```python
from build123d import *

# Parameters (mm, degrees)
F0_W     = 100
F0_H     = 100
F1_DEPTH = 10
F2_SIZE  = 12
F4_D     = 9.5


with BuildPart() as f1:
    # F0 (on Top) → F1 (new body)
    with BuildSketch(Plane.XY):
        Rectangle(F0_W, F0_H)
    extrude(amount=F1_DEPTH)

    # F2
    f2_edges = [f1.edges().sort_by_distance(p)[0] for p in [
        (50, -50, 5),
        (50, 50, 5),
        (-50, -50, 5),
        (-50, 50, 5),
    ]]
    chamfer(f2_edges, length=F2_SIZE)

    # F4 (through all)
    with Locations(Plane.XY.offset(10)):
        with Locations((-15.5, 0), (-34, 0), (-34, -27.5), (-34, 27.5), (34, 27.5), (34, 0), (34, -27.5), (0, 0)):
            Hole(F4_D / 2)


solid = f1.part
```
Read the model definition and answer for the solid it produces. Units are mm, in the model's axes. Give positions to 0.01 mm unless a question says otherwise; leave off trailing zeros. Write each loop counter-clockwise with the first axis right and the second up, starting at its lowest first coordinate (ties: lowest second). Pieces come first, ordered by that corner, then holes. Notation, with made-up numbers: (-19, 24) -> (-11, 24) arc R17 cw to (-11, 51) -> close; hole circle Ø9 at (43.5, 69). An arc over 180 degrees is marked (long way). Answer in a Markdown table with one row per item.
1) This flat-tipped pin is pushed along its axis until it touches: pin 1 Ø8.5 at (x, y) = (0, 0) entering from +Z. Where does it stop, or does it pass through?
Results list:
| item | result |
|---|---|
| pin 1 | through |
2) Section B-B on x = -15.5 is taken. Give the vertices of the cut face in (y, z).
Results list:
| item | result |
|---|---|
| outline | (-50, 0) -> (-4.75, 0) -> (-4.75, 10) -> (-50, 10) -> close; (4.75, 0) -> (50, 0) -> (50, 10) -> (4.75, 10) -> close |
3) Section D-D on z = 8.25 is taken. Count the separate pieces of the cut face and the enclosed holes in it, plus the area to 3 significant figures.
Results list:
| item | result |
|---|---|
| separate pieces | 1 |
| enclosed holes | 8 |
| area | 9,140 mm^2 |
4) Determine the mould class of faces 1 (the flat face through (-44, -44, 5)), 2 (the flat face through (-1, 50, 5)), 3 (the flat face through (10, 1, 10)), 4 (the cylindrical face through (29.612, -1.819, 4.93)) for opening direction Y: released by +Y, released by -Y, zero draft, split by the parting line, or undercut.
Results list:
| item | result |
|---|---|
| face 1 | released by -Y |
| face 2 | released by +Y |
| face 3 | zero draft |
| face 4 | undercut |
5) Section A-A on y = 0 is taken. Give the vertices of the cut face in (x, z).
Results list:
| item | result |
|---|---|
| outline | (-50, 0) -> (-38.75, 0) -> (-38.75, 10) -> (-50, 10) -> close; (-29.25, 0) -> (-20.25, 0) -> (-20.25, 10) -> (-29.25, 10) -> close; (-10.75, 0) -> (-4.75, 0) -> (-4.75, 10) -> (-10.75, 10) -> close; (4.75, 0) -> (29.25, 0) -> (29.25, 10) -> (4.75, 10) -> close; (38.75, 0) -> (50, 0) -> (50, 10) -> (38.75, 10) -> close |
6) Section C-C on y = -27.5 is taken. Give the vertices of the cut face in (x, z).
Results list:
| item | result |
|---|---|
| outline | (-50, 0) -> (-38.75, 0) -> (-38.75, 10) -> (-50, 10) -> close; (-29.25, 0) -> (29.25, 0) -> (29.25, 10) -> (-29.25, 10) -> close; (38.75, 0) -> (50, 0) -> (50, 10) -> (38.75, 10) -> close |
7) Straight lines are drawn through the part: line 1 (Y direction, x = -34, z = 6); line 2 (Y direction, x = -31, z = 8.75); line 3 (X direction, y = -24, z = 3). For each, find the intervals that lie inside material, in ascending order. Write a range as [from, to].
Results list:
| item | result |
|---|---|
| line 1 | [-50, -32.25], [-22.75, -4.75], [4.75, 22.75], [32.25, 50] |
| line 2 | [-50, -31.18], [-23.82, -3.68], [3.68, 23.82], [31.18, 50] |
| line 3 | [-50, -37.21], [-30.79, 30.79], [37.21, 50] |
